Model file for the job. Use its own axes, mm. A direction names the side the tool comes from. Give positions to 0.01 mm unless a question says otherwise; leave off trailing zeros. Loops run counter-clockwise (first coordinate to the right, second up) from the corner with the lowest first, then second, coordinate; pieces in that order, holes last. Notation, with made-up numbers: M -19,-18 L 14,-18 A36 ccw 14,19 Z; hole C -12.5,83.5 d5. An arc over 180 degrees is marked long. Use CSV: the item, a comma, the result in double quotes. Start each with the question number.
(1) Slice it at B-B on x = 237. List the corners of the cut face in (y, z), and give its area (3 significant figures).
(2) Flat gauge pins, fed straight in: P1, Ø4, axis at x = -77, z = 346.5, coming from the -Y side; P2, Ø12, axis at y = -16.5, z = -23, coming from the -X side; P3, Ø20, axis at x = 187, y = -18, coming from the -Z side. Where does each tip first touch, or does it go through?
(3) Slice it at C-C on z = -128.5. List the corners of the cut face in (x, y), and give its area (3 significant figures).
(4) Tool access for faces 1 (the face through (-6, 436, -425)), 2 (the face through (500, 444, 7)), 3 (the face through (-7, -20, 465)), 4 (the face through (-500, 444, 7)), 5 (the face through (-7, -20, -465)): list every direction of +Z, -Z, +X, -X, +Y, -Y with a clear straight run to the whole face (end or side of a thin tool).
(5) Two-plate mould, pull along X, no slides. Class faces 6 (the face through (425, 436, 6)), 7 (the face through (465, -20, 7)), 8 (the face through (-465, -20, 7)), 9 (the face through (-7, 900, -7)): pulls with the +X half, pulls with the -X half, needs draft (parallel to the pull), parting line crosses it, or undercut.
(6) Wall check: line 1 along Z through (x, y) = (137.5, 276.5); line 2 along Y through (x, z) = (151, 368.5). Give the ranges that are in metal, low to high. Write a range as from..to.
(7) Slice it at A-A on y = 433.5. List the corners of the cut face in (x, z).
```python
from build123d import *

# Parameters (mm, degrees)
SKETCH1_W           = 1000
SKETCH1_H           = 1000
SKETCH1_W_2         = 930
SKETCH1_H_2         = 930
SKETCH1_W_3         = 850
SKETCH1_H_3         = 850
BOSS_EXTRUDE2_DEPTH = 900
SKETCH1_4_W         = 930
SKETCH1_4_H         = 930
SKETCH1_4_W_2       = 850
SKETCH1_4_H_2       = 850
BOSS_EXTRUDE3_DEPTH = 40
BOSS_EXTRUDE4_START = 900
SKETCH1_5_W         = 850
SKETCH1_5_H         = 850
BOSS_EXTRUDE4_DEPTH = 2


with BuildPart() as part:
    # Sketch1 → Boss-Extrude2 (new body)
    # profile 1 of 2: a face of its own
    with BuildSketch(Plane(origin=(0, 0, 0), x_dir=(1, 0, 0), z_dir=(0, 1, 0))):
        Rectangle(SKETCH1_W, SKETCH1_H)
        Rectangle(SKETCH1_W_2, SKETCH1_H_2, mode=Mode.SUBTRACT)
    # profile 2 of 2: a face of its own
    with BuildSketch(Plane(origin=(0, 0, 0), x_dir=(1, 0, 0), z_dir=(0, 1, 0))):
        Rectangle(SKETCH1_W_2, SKETCH1_H_2)
        Rectangle(SKETCH1_W_3, SKETCH1_H_3, mode=Mode.SUBTRACT)
    extrude(amount=BOSS_EXTRUDE2_DEPTH)

    # Sketch1<4> → Boss-Extrude3 (add)
    with BuildSketch(Plane(origin=(0, 0, 0), x_dir=(1, 0, 0), z_dir=(0, 1, 0))):
        Rectangle(SKETCH1_4_W, SKETCH1_4_H)
        Rectangle(SKETCH1_4_W_2, SKETCH1_4_H_2, mode=Mode.SUBTRACT)
    extrude(amount=-BOSS_EXTRUDE3_DEPTH)

    # Sketch1<5> → Boss-Extrude4 (add)
    with BuildSketch(Plane(origin=(0, 0, 0), x_dir=(1, 0, 0), z_dir=(0, 1, 0)).offset(BOSS_EXTRUDE4_START)):
        Rectangle(SKETCH1_5_W, SKETCH1_5_H)
    extrude(amount=-BOSS_EXTRUDE4_DEPTH)


solid = part.part
```
Reply:
1,outline,"M -40,-465 L 0,-465 L 0,-500 L 900,-500 L 900,500 L 0,500 L 0,465 L -40,465 L -40,425 L 898,425 L 898,-425 L -40,-425 Z"
1,area,"140,000 mm^2"
2,P1,"stops at y = 898"
2,P2,"stops at x = -465"
2,P3,"stops at z = -465"
3,outline,"M -500,0 L -465,0 L -465,-40 L -425,-40 L -425,898 L 425,898 L 425,-40 L 465,-40 L 465,0 L 500,0 L 500,900 L -500,900 Z"
3,area,"140,000 mm^2"
4,face 1,"-Y"
4,face 2,"+Z, -Z, +X, +Y, -Y"
4,face 3,"+Z, +X, -X, -Y"
4,face 4,"+Z, -Z, -X, +Y, -Y"
4,face 5,"-Z, +X, -X, -Y"
5,face 6,"undercut"
5,face 7,"pulls with the +X half"
5,face 8,"pulls with the -X half"
5,face 9,"needs draft"
6,line 1,"z = -500..-425, 425..500"
6,line 2,"y = 898..900"
7,outline,"M -500,-500 L 500,-500 L 500,500 L -500,500 Z; hole M -425,-425 L 425,-425 L 425,425 L -425,425 Z"
